Geometry check sheet. Reference: the model listing, model coordinates, mm. Face numbers are marked on the shaded views. A direction names the side the tool comes from. Give positions to 0.01 mm unless a question says otherwise; leave off trailing zeros. Loops run counter-clockwise (first coordinate to the right, second up) from the corner with the lowest first, then second, coordinate; pieces in that order, holes last. Notation, with made-up numbers: (-29, 13) -> (-2, 13) arc R19 ccw to (-2, 31) -> close; hole circle Ø10 at (-14, -18). An arc over 180 degrees is marked (long way). Write item = value, one per line.
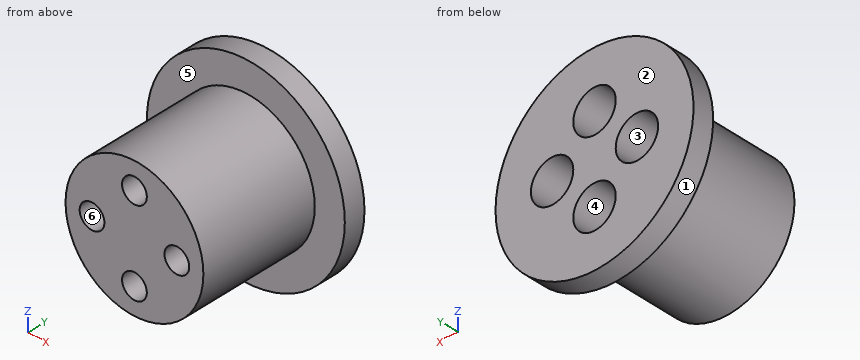
```python
from build123d import *

# Parameters (mm, degrees)
SKETCH1_R           = 9.75
BOSS_EXTRUDE1_DEPTH = 17
SKETCH2_R           = 14
BOSS_EXTRUDE2_DEPTH = 3
SKETCH3_R           = 1.75
CUT_EXTRUDE1_DEPTH  = 21
CIRPATTERN1_COUNT   = 4
SKETCH4_R           = 3
CUT_EXTRUDE2_DEPTH  = 10
CIRPATTERN2_COUNT   = 4


with BuildPart() as part:
    # Sketch1 → Boss-Extrude1 (new body)
    with BuildSketch(Plane(origin=(0, 0, 0), x_dir=(1, 0, 0), z_dir=(0, 1, 0))):
        Circle(SKETCH1_R)
    extrude(amount=BOSS_EXTRUDE1_DEPTH)

    # Sketch2 → Boss-Extrude2 (add)
    with BuildSketch(Plane(origin=(0, 17, 0), x_dir=(1, 0, 0), z_dir=(0, 1, 0))):
        Circle(SKETCH2_R)
    extrude(amount=BOSS_EXTRUDE2_DEPTH)

    # Sketch3 → Cut-Extrude1 (cut, through all)
    with BuildSketch(Plane.XZ):
        with Locations((0, 6)):
            Circle(SKETCH3_R)
    cut_extrude1 = extrude(amount=-CUT_EXTRUDE1_DEPTH, mode=Mode.SUBTRACT)

    # CirPattern1: Cut-Extrude1 ×4 about axis
    cirpattern1_axis = Axis((0, 0, 0), (0, 1, 0))
    for i in range(1, CIRPATTERN1_COUNT):
        add(cut_extrude1.rotate(cirpattern1_axis, i * 360 / CIRPATTERN1_COUNT), mode=Mode.SUBTRACT)

    # Sketch4 → Cut-Extrude2 (cut)
    with BuildSketch(Plane(origin=(0, 20, 0), x_dir=(1, 0, 0), z_dir=(0, 1, 0))):
        with Locations((0, 6)):
            Circle(SKETCH4_R)
    cut_extrude2 = extrude(amount=-CUT_EXTRUDE2_DEPTH, mode=Mode.SUBTRACT)

    # CirPattern2: Cut-Extrude2 ×4 about axis
    cirpattern2_axis = Axis((0, 0, 0), (0, 1, 0))
    for i in range(1, CIRPATTERN2_COUNT):
        add(cut_extrude2.rotate(cirpattern2_axis, i * 360 / CIRPATTERN2_COUNT), mode=Mode.SUBTRACT)


solid = part.part
```
Item 1: Gauge pin test, flat ends, axial feed: pin 1 (3 mm diameter, centred on x = 0, z = -6, fed in from -Y); pin 2 (1.5 mm diameter, centred on x = -6, y = 2.5, fed in from -Z); pin 3 (12 mm diameter, centred on y = 15.5, z = -10, fed in from -X); pin 4 (4 mm diameter, centred on x = 7, y = 8.5, fed in from -Z). Record the tip position at first contact, or that the pin passes through.
Answer:
pin_1 = through
pin_2 = -8.22
pin_3 = -13.36
pin_4 = -8.37
Item 2: Section check D-D, the plane y = 2.25. Record the cut outline in (x, z), plus the area to 3 significant figures.
Answer:
outline = circle Ø19.5 at (0, 0); hole circle Ø3.5 at (-6, 0); hole circle Ø3.5 at (0, -6); hole circle Ø3.5 at (0, 6); hole circle Ø3.5 at (6, 0)
area = 260 mm^2
Item 3: Section check A-A, the plane z = 0. Record the cut outline in (x, y), plus the area to 4 significant figures.
Answer:
outline = (-14, 17) -> (-9.75, 17) -> (-9.75, 0) -> (-7.75, 0) -> (-7.75, 10) -> (-9, 10) -> (-9, 20) -> (-14, 20) -> close; (-4.25, 0) -> (4.25, 0) -> (4.25, 10) -> (3, 10) -> (3, 20) -> (-3, 20) -> (-3, 10) -> (-4.25, 10) -> close; (7.75, 0) -> (9.75, 0) -> (9.75, 17) -> (14, 17) -> (14, 20) -> (9, 20) -> (9, 10) -> (7.75, 10) -> close
area = 225.5 mm^2
Item 4: Draft check along X on the marked faces 1, 2 and 3. Enter one of: +X half, -X half, draft (parallel to the pull), parting line (faces both ways), or undercut.
Answer:
face_1 = parting line
face_2 = draft
face_3 = undercut
Item 5: Section check C-C, the plane z = 6.75. Record the cut outline in (x, y), plus the area to 3 significant figures.
Answer:
outline = (-12.27, 17) -> (-7.04, 17) -> (-7.04, 0) -> (-1.58, 0) -> (-1.58, 10) -> (-2.9, 10) -> (-2.9, 20) -> (-12.27, 20) -> close; (1.58, 0) -> (7.04, 0) -> (7.04, 17) -> (12.27, 17) -> (12.27, 20) -> (2.9, 20) -> (2.9, 10) -> (1.58, 10) -> close
area = 223 mm^2
Item 6: Thickness scan on L1, parallel to Z at x = 0, y = 7.25; L2, parallel to X at y = 16, z = 0; L3, parallel to X at y = 18, z = 0. Record the ranges inside material, lowest first. Write a range as [from, to].
Answer:
L1 = [-9.75, -7.75], [-4.25, 4.25], [7.75, 9.75]
L2 = [-9.75, -9], [-3, 3], [9, 9.75]
L3 = [-14, -9], [-3, 3], [9, 14]
Item 7: Tool access check on the marked faces 4, 5 and 6. Record the directions out of +Z, -Z, +X, -X, +Y, -Y that give a thin tool (end or side, any length) a straight path to the whole face; none if there is none.
Answer:
face_4 = +Y
face_5 = -Y
face_6 = +Y, -Y
Item 8: Section check B-B, the plane x = 0. Record the cut outline in (y, z).
Answer:
outline = (0, -9.75) -> (17, -9.75) -> (17, -14) -> (20, -14) -> (20, -9) -> (10, -9) -> (10, -7.75) -> (0, -7.75) -> close; (0, -4.25) -> (10, -4.25) -> (10, -3) -> (20, -3) -> (20, 3) -> (10, 3) -> (10, 4.25) -> (0, 4.25) -> close; (0, 7.75) -> (10, 7.75) -> (10, 9) -> (20, 9) -> (20, 14) -> (17, 14) -> (17, 9.75) -> (0, 9.75) -> close
